Autodesk Inventor part; units mm, degrees
ref_plane "YZ Plane" through (0, 0, 0) normal (1, 0, 0) x (0, 1, 0)
ref_plane "XZ Plane" through (0, 0, 0) normal (0, 1, 0) x (-1, 0, 0)
ref_plane "XY Plane" through (0, 0, 0) normal (0, 0, 1) x (1, 0, 0)
sketch "Sketch1" plane through (0, 0, 0) normal (0, 1, 0) x (-1, 0, 0)
  line L0 (0, 0) -> (-30, 0) construction
  line L1 (0, 25) -> (-30, 25)
  line L2 (-30, -25) -> (0, -25)
  arc A0 (0, -25) -> (0, 25) centre (0, 0) ccw
  arc A1 (-30, 25) -> (-30, -25) centre (-30, 0) ccw
  circle A2 centre (8, 0) radius 2.45
  line L3 (0, 0) -> (25, 0) construction
  circle A3 centre (8, 0) radius 22.5 construction
  circle A4 centre (8, 0) radius 15 construction
  point P0 (-15, 0)
  dimension "d26" = 50
  dimension "d27" = 30
  dimension "d28" = 4.9
  dimension "d29" = 8
  dimension "d30" = 17
  dimension "d31" = 45
  dimension "d32" = 30
extrude "Extrusion6" add sketch "Sketch1" along normal blind 19.2
equation "\"d23\" = printing_w"
equation "\"blade_w\" = 0.3"
equation "\"calib_w\" = 0.3"
equation "\"print_fit_w\" = 0.2"
equation "\"printing_w\" = -calib_w + nominal_w - blade_w - print_fit_w"
properties part number "071_0202_RollCutter20mmCenter"
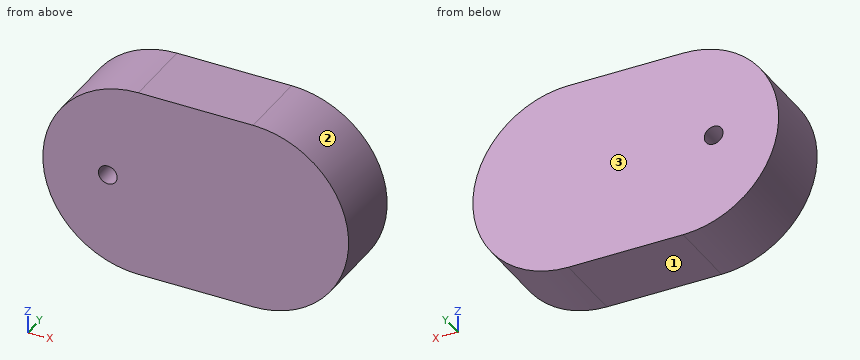
Here's how the part is built. I have some questions about the finished solid (model axes, mm). Face numbers are marked on the shaded views. Give positions to 0.01 mm unless a question says otherwise; leave off trailing zeros. Loops run counter-clockwise (first coordinate to the right, second up) from the corner with the lowest first, then second, coordinate; pieces in that order, holes last. Notation, with made-up numbers: M 40,75 L 44,75 A27 ccw 44,113 Z; hole C 89.25,71.25 d7. An arc over 180 degrees is marked long. Put each result on its own line as item: value. Start each with the question number.
(1) I want a section at A-A on z = 0. Please give me the cut outline in (x, y).
(2) I want a section at D-D on z = -14. Please give me the cut outline in (x, y).
(3) I need wall thicknesses on line 1 along Z through (x, y) = (-8, 5.75); line 2 along X through (y, z) = (13, -4); line 3 along X through (y, z) = (6, 13). Which ranges of each line are inside material? Lowest first, please. Write a range as [from, to].
(4) I want a section at C-C on y = 17.25. Please give me the cut outline in (x, z), then the cut area to 3 significant figures.
(5) If we mould it in two halves opening along Z, with no side actions, what happens to the marked faces 1, 2 and 3? For each: +Z half, -Z half, draft (parallel to the pull), parting line (faces both ways), or undercut.
(6) Will these pins go through, and if not, where does the flat tip stop? pin 1 Ø1 at (y, z) = (5, 13) entering from -X; pin 2 Ø6 at (x, y) = (43.5, 11.5) entering from +Z; pin 3 Ø1 at (x, y) = (46, 4) entering from +Z; pin 4 Ø5.5 at (x, z) = (-8, 0) entering from +Y.
(7) I want a section at B-B on x = -8.5. Please give me the cut outline in (y, z), then the cut area to 3 significant figures.
Answer block:
1. outline: M -25,0 L -10.45,0 L -10.45,19.2 L -25,19.2 Z; M -5.55,0 L 55,0 L 55,19.2 L -5.55,19.2 Z
2. outline: M -20.71,0 L 50.71,0 L 50.71,19.2 L -20.71,19.2 Z
3. line 1: [-23.69, -2.45], [2.45, 23.69]
3. line 2: [-24.68, 54.68]
3. line 3: [-21.35, 51.35]
4. outline: M 0,-25 L 30,-25 A25 ccw 30,25 L 0,25 A25 ccw Z; hole C -8,0 d4.9
4. area: 3,440 mm^2
5. face 1: -Z half
5. face 2: parting line
5. face 3: draft
6. pin 1: x = -21.65
6. pin 2: z = 22.69
6. pin 3: z = 19.62
6. pin 4: y = 19.2
7. outline: M 0,-23.51 L 19.2,-23.51 L 19.2,-2.4 L 0,-2.4 Z; M 0,2.4 L 19.2,2.4 L 19.2,23.51 L 0,23.51 Z
7. area: 811 mm^2
